```python
from build123d import *

# Parameters (mm, degrees)
F0_W          = 114.3
F0_H          = 110.8363599028
F2_DEPTH      = 2
F1_E1_W       = 13.8702858239
F1_E1_H       = 35.56
F3_DEPTH      = 2
F5_E4_W       = 13.8702858239
F5_E4_H       = 20
F6_DEPTH      = 2
F7_R          = 1.905
F8_DEPTH      = 6.858
F8_DEPTH_BACK = 2.032


with BuildPart() as f2:
    # F0 (on Top) → F2 (new body)
    with BuildSketch(Plane.XY):
        Rectangle(F0_W, F0_H)
    extrude(amount=F2_DEPTH)

    # F1_E1 (on explicit) → F3 (join)
    with BuildSketch(Plane(origin=(-8.9655527845, 33.3296358585, 0), x_dir=(1, 0, 0), z_dir=(0, -1, 0))):
        with Locations((6.935142912, 17.78)):
            Rectangle(F1_E1_W, F1_E1_H)
    extrude(amount=F3_DEPTH)

    # F5_E4 (on explicit) → F6 (join)
    with BuildSketch(Plane(origin=(-8.9655527845, 31.3296358585, 35.56), x_dir=(1, 0, 0), z_dir=(0, 0, -1))):
        with Locations((6.935142912, 10)):
            Rectangle(F5_E4_W, F5_E4_H)
    extrude(amount=F6_DEPTH)

    # F7 (on face) → F8 (cut, two sides)
    with BuildSketch(Plane(origin=(0, 0, 35.56), x_dir=(1, 0, 0), z_dir=(0, 0, -1))) as f8_sk:
        with Locations((-1.9456632435, -20.2625636011)):
            Circle(F7_R)
    extrude(amount=F8_DEPTH, mode=Mode.SUBTRACT)
    extrude(f8_sk.sketch, amount=-F8_DEPTH_BACK, mode=Mode.SUBTRACT)


solid = f2.part
```
The model under review builds one solid part; all positions refer to its coordinate system, in mm. A direction names the side the tool comes from. Round coordinates to 2 decimals unless told otherwise and drop trailing zeros. Order: outer loops, then holes, each group sorted by start corner. A loop starts at its lowest first (then second) coordinate and runs counter-clockwise, first axis right, second up. Notation, with made-up numbers: (89, 37) - (125, 37) arc R28 ccw to (125, 66) - close; hole circle Ø11 at (70, 69). An arc over 180 degrees is marked (long way). Answer in a Markdown table with one row per item.
(1) Take a section at B-B on x = 44. Write out the cut boundary in (y, z), plus the area to 3 significant figures.
Result set:
| item | result |
|---|---|
| outline | (-55.42, 0) - (55.42, 0) - (55.42, 2) - (-55.42, 2) - close |
| area | 222 mm2 |
(2) Take a section at A-A on y = 29.5. Write out the cut boundary in (x, z).
Result set:
| item | result |
|---|---|
| outline | (-57.15, 0) - (57.15, 0) - (57.15, 2) - (-57.15, 2) - close; (-8.97, 33.56) - (4.9, 33.56) - (4.9, 35.56) - (-8.97, 35.56) - close |
(3) Take a section at C-C on z = 19. Write out the cut boundary in (x, y), plus the area to 3 significant figures.
Result set:
| item | result |
|---|---|
| outline | (-8.97, 31.33) - (4.9, 31.33) - (4.9, 33.33) - (-8.97, 33.33) - close |
| area | 27.7 mm2 |
(4) Mouldability with a two-part tool opening along Z and no side actions: class faces 1 (the face through (-8.966, 32, 24)), 2 (the face through (-2, 31.33, 18)), 3 (the face through (-4, 21, 33.56)), 4 (the face through (-1, 1, 0)) as released by +Z, released by -Z, zero draft, split by the parting line, or undercut.
Result set:
| item | result |
|---|---|
| face 1 | zero draft |
| face 2 | undercut |
| face 3 | undercut |
| face 4 | released by -Z |
(5) For line 1 (Z direction, x = -24.5, y = -28.5); line 2 (Y direction, x = -6, z = 32), list the stretches that pass through material, from the lowest coordinate up. Write a range as from..to.
Result set:
| item | result |
|---|---|
| line 1 | z = 0..2 |
| line 2 | y = 31.33..33.33 |
(6) Clearance check with flat-ended pins moving along their axes: P1, Ø1, axis at x = 30, y = 36, coming from the +Z side; P2, Ø4, axis at x = 0.5, z = 17.5, coming from the -Y side; P3, Ø6.5, axis at y = 26.5, z = 23.5, coming from the +X side; P4, Ø11, axis at x = 0.5, z = 17.5, coming from the +Y side. State where each tip first meets the part, or that it passes through.
Result set:
| item | result |
|---|---|
| P1 | stops at z = 2 |
| P2 | stops at y = 31.33 |
| P3 | passes through |
| P4 | stops at y = 33.33 |
(7) Machinability: for faces 5 (the face through (-2.36, 22.12, 34.57)), 6 (the face through (4.905, 32, 24)), 7 (the face through (-2, 33.33, 19)), which of the approach directions +Z, -Z, +X, -X, +Y, -Y give a long, thin tool a straight path to every point of the face, cutting with its end or side? Answer none if there is none.
Result set:
| item | result |
|---|---|
| face 5 | +Z |
| face 6 | +Z, +X, +Y, -Y |
| face 7 | +Z, +X, -X, +Y |
